```python
from build123d import *

# Parameters (mm, degrees)
SKETCH1_W           = 30
SKETCH1_H           = 60
BOSS_EXTRUDE1_DEPTH = 10
SKETCH2_W           = 10
SKETCH2_H           = 60
BOSS_EXTRUDE2_DEPTH = 50
SKETCH3_R           = 2
CUT_EXTRUDE1_DEPTH  = 50
SKETCH4_W           = 10
SKETCH4_H           = 20
CUT_EXTRUDE2_DEPTH  = 50


with BuildPart() as part:
    # Sketch1 → Boss-Extrude1 (new body)
    with BuildSketch(Plane.XY):
        with Locations((18.070175439, 2.280701754)):
            Rectangle(SKETCH1_W, SKETCH1_H)
    extrude(amount=BOSS_EXTRUDE1_DEPTH)

    # Sketch2 → Boss-Extrude2 (add)
    with BuildSketch(Plane.XY.offset(10)):
        with Locations((28.070175439, 2.280701754)):
            Rectangle(SKETCH2_W, SKETCH2_H)
    extrude(amount=BOSS_EXTRUDE2_DEPTH)

    # Sketch3 → Cut-Extrude1 (cut)
    with BuildSketch(Plane.XY.offset(10)):
        with Locations((13.070175439, 22.280701754)):
            Circle(SKETCH3_R)
        with Locations((13.070175439, 2.280701754)):
            Circle(SKETCH3_R)
    extrude(amount=-CUT_EXTRUDE1_DEPTH, mode=Mode.SUBTRACT)

    # Sketch4 → Cut-Extrude2 (cut)
    with BuildSketch(Plane(origin=(0, 0, 0), x_dir=(-1, 0, 0), z_dir=(0, 0, -1))):
        with Locations((-28.070175439, 2.280701754)):
            Rectangle(SKETCH4_W, SKETCH4_H)
    extrude(amount=-CUT_EXTRUDE2_DEPTH, mode=Mode.SUBTRACT)


solid = part.part
```
CAD build for the part. Positions are in the model's coordinates, mm. A direction names the side the tool comes from. Round coordinates to 2 decimals unless told otherwise and drop trailing zeros. Write each loop counter-clockwise with the first axis right and the second up, starting at its lowest first coordinate (ties: lowest second). Pieces come first, ordered by that corner, then holes. Notation, with made-up numbers: (19, 40) -> (63, 40) arc R29 cw to (63, 74) -> close; hole circle Ø1 at (15, 6.5). An arc over 180 degrees is marked (long way). Answer in a Markdown table with one row per item. Add a question column.
Item 1: Mould opens along Y. For faces 5 (the face through (25, 32.281, 23)), 6 (the face through (25, -27.719, 23)), 7 (the face through (13.993, 20.506, 5.07)), 8 (the face through (23.07, -11, 35)) say: pulls with the +Y half, pulls with the -Y half, needs draft (parallel to the pull), parting line crosses it, or undercut.
Item 2: Saw through at C-C, the plane x = 13.5. Write the cut outline in (y, z).
Item 3: Drop flat-ended pins along their axis: pin 1 Ø5 at (y, z) = (-2.5, 5.5) entering from +X; pin 2 Ø5 at (x, y) = (28.5, 7) entering from -Z; pin 3 Ø8 at (y, z) = (11, 28.5) entering from -X. Give the stop position or say it passes through.
Item 4: Saw through at A-A, the plane y = -5. Write the cut outline in (x, z).
Item 5: Which spindle directions (+Z, -Z, +X, -X, +Y, -Y) get a long thin tool onto all of the face, cutting with end or side? Do faces 1 (the face through (11, 3, 10)), 2 (the face through (18, 3, 0)), 3 (the face through (28, 12.281, 25)), 4 (the face through (28, 2, 50)). Say none if no direction does.
Item 6: Saw through at B-B, the plane z = 25.5. Write the cut outline in (x, y).
Item 7: Saw through at D-D, the plane z = 6. Write the cut outline in (x, y), then the cut area to 3 significant figures.
Item 8: Drill centre lines: line 1 (Y direction, x = 27, z = 18); line 2 (Z direction, x = 21, y = 29); line 3 (Z direction, x = 23.75, y = 3.5). Where is each one in solid material? Low to high. Write a range as from..to.
Findings below:
| question | item | result |
|---|---|---|
| 1 | face 5 | pulls with the +Y half |
| 1 | face 6 | pulls with the -Y half |
| 1 | face 7 | undercut |
| 1 | face 8 | needs draft |
| 2 | outline | (-27.72, 0) -> (0.33, 0) -> (0.33, 10) -> (-27.72, 10) -> close; (4.23, 0) -> (20.33, 0) -> (20.33, 10) -> (4.23, 10) -> close; (24.23, 0) -> (32.28, 0) -> (32.28, 10) -> (24.23, 10) -> close |
| 3 | pin 1 | stops at x = 23.07 |
| 3 | pin 2 | stops at z = 50 |
| 3 | pin 3 | stops at x = 23.07 |
| 4 | outline | (3.07, 0) -> (23.07, 0) -> (23.07, 10) -> (3.07, 10) -> close; (23.07, 50) -> (33.07, 50) -> (33.07, 60) -> (23.07, 60) -> close |
| 5 | face 1 | +Z, -X, +Y, -Y |
| 5 | face 2 | -Z, +X, -X, +Y, -Y |
| 5 | face 3 | -Z, +X |
| 5 | face 4 | -Z, +X, -X |
| 6 | outline | (23.07, -27.72) -> (33.07, -27.72) -> (33.07, -7.72) -> (23.07, -7.72) -> close; (23.07, 12.28) -> (33.07, 12.28) -> (33.07, 32.28) -> (23.07, 32.28) -> close |
| 7 | outline | (3.07, -27.72) -> (33.07, -27.72) -> (33.07, -7.72) -> (23.07, -7.72) -> (23.07, 12.28) -> (33.07, 12.28) -> (33.07, 32.28) -> (3.07, 32.28) -> close; hole circle Ø4 at (13.07, 2.28); hole circle Ø4 at (13.07, 22.28) |
| 7 | area | 1,570 mm^2 |
| 8 | line 1 | y = -27.72..-7.72, 12.28..32.28 |
| 8 | line 2 | z = 0..10 |
| 8 | line 3 | z = 50..60 |
